```python
from build123d import *

# Parameters (mm, degrees)
BOSS_EXTRUDE1_DEPTH     = 6.35
FILLET1_R               = 6.35
F_1_4_CLEARANCE_HOLE2_D = 6.7564
F_8_CLEARANCE_HOLE1_D   = 4.4958


with BuildPart() as part:
    # Sketch1 → Boss-Extrude1 (new body)
    with BuildSketch(Plane(origin=(0, 0, 0), x_dir=(1, 0, 0), z_dir=(0, 1, 0))):
        Polygon((-26.866954165, 159.9), (-52.809618943, 159.9), (-99.343756128, 133.03350337), (-59.901828464, 64.718080709), (20.2, 64.718080709), (20.2, 128.218080709), (-8.575389533, 128.218080709), align=None)
    extrude(amount=-BOSS_EXTRUDE1_DEPTH)

    # Fillet1
    fillet1_edges = [part.edges().sort_by_distance(p)[0] for p in [
        (-52.809618943, -3.175, -159.9),
        (-26.866954165, -3.175, -159.9),
        (-8.575389533, -3.175, -128.218080709),
        (20.2, -3.175, -128.218080709),
        (20.2, -3.175, -64.718080709),
        (-59.901828464, -3.175, -64.718080709),
        (-99.343756128, -3.175, -133.03350337),
    ]]
    fillet(fillet1_edges, radius=FILLET1_R)

    # 1/4 Clearance Hole2 (through all)
    with Locations(Plane(origin=(0, -6.35, 0), x_dir=(-1, 0, 0), z_dir=(0, -1, 0))):
        with Locations((87.344864157, 131.300812842), (33.535349774, 152.4), (-12.58, 74.243080709), (-12.58, 118.693080709)):
            Hole(F_1_4_CLEARANCE_HOLE2_D / 2)

    # #8 Clearance Hole1 (through all)
    with Locations(Plane(origin=(0, 0, 0), x_dir=(1, 0, 0), z_dir=(0, 1, 0))):
        with Locations((-54.269039573, 121.866162864), (-28.872875262, 96.469998554)):
            Hole(F_8_CLEARANCE_HOLE1_D / 2)


solid = part.part
```
The model under review builds one solid part; all positions refer to its coordinate system, in mm. A direction names the side the tool comes from. Give positions to 0.01 mm unless a question says otherwise; leave off trailing zeros. Write each loop counter-clockwise with the first axis right and the second up, starting at its lowest first coordinate (ties: lowest second). Pieces come first, ordered by that corner, then holes. Notation, with made-up numbers: M 20.25,0 L 61.25,0 A19 cw 61.25,7 Z; hole C 58,42 d7. An arc over 180 degrees is marked long. Answer in a Markdown table with one row per item.
Item 1: Tool access review of faces 4 (the face through (-53.976, -3.219, -124.095)), 5 (the face through (5, -3, -128.218)): name each direction out of +Z, -Z, +X, -X, +Y, -Y from which nothing blocks a thin tool from reaching the whole face with its end or side.
Check sheet entries:
| item | result |
|---|---|
| face 4 | +Y, -Y |
| face 5 | -Z, +X, +Y, -Y |
Item 2: For line 1 along Z through (x, y) = (12.58, -3.25); line 2 along Z through (x, y) = (-55.5, -3.25); line 3 along X through (y, z) = (-4, -129.5), list the stretches that pass through material, from the lowest coordinate up.
Check sheet entries:
| item | result |
|---|---|
| line 1 | -128.22 to -122.07, -115.31 to -77.62, -70.86 to -64.72 |
| line 2 | -158.35 to -123.75, -119.99 to -64.72 |
| line 3 | -96.9 to -90.2, -84.49 to -8.74 |
Item 3: Draft analysis for pull direction X (two halves, no side actions). For faces 1 (the face through (-17.62, -3.13, -143.88)), 2 (the face through (-27.09, -3.22, -95.1)), 3 (the face through (-73.787, -3.131, -147.789)), state which applies: +X half, -X half, draft (parallel to the pull), parting line (faces both ways), or undercut.
Check sheet entries:
| item | result |
|---|---|
| face 1 | +X half |
| face 2 | undercut |
| face 3 | -X half |
Item 4: Add section A-A on x = 12.58. Give the boundary of the cut face in (y, z).
Check sheet entries:
| item | result |
|---|---|
| outline | M -6.35,-128.22 L 0,-128.22 L 0,-122.07 L -6.35,-122.07 Z; M -6.35,-115.31 L 0,-115.31 L 0,-77.62 L -6.35,-77.62 Z; M -6.35,-70.86 L 0,-70.86 L 0,-64.72 L -6.35,-64.72 Z |
Item 5: Add section D-D on x = -3. Give the boundary of the cut face in (y, z).
Check sheet entries:
| item | result |
|---|---|
| outline | M -6.35,-128.22 L 0,-128.22 L 0,-64.72 L -6.35,-64.72 Z |
Item 6: Add section C-C on y = -3. State how many separate pieces and enclosed holes the cut face has, plus the area to 3 significant figures.
Check sheet entries:
| item | result |
|---|---|
| separate pieces | 1 |
| enclosed holes | 6 |
| area | 8,000 mm2 |
Item 7: For P1, Ø3, axis at x = 7, y = -2.5, coming from the -Z side; P2, Ø1.5, axis at y = -4, z = -121.5, coming from the -X side, all flat-tipped, find the tip position at first contact; note any pin that passes through.
Check sheet entries:
| item | result |
|---|---|
| P1 | z = -128.22 |
| P2 | x = -93.12 |
Item 8: Add section B-B on z = -152.4. Give the boundary of the cut face in (x, y).
Check sheet entries:
| item | result |
|---|---|
| outline | M -65.8,-6.35 L -36.91,-6.35 L -36.91,0 L -65.8,0 Z; M -30.16,-6.35 L -22.54,-6.35 L -22.54,0 L -30.16,0 Z |
